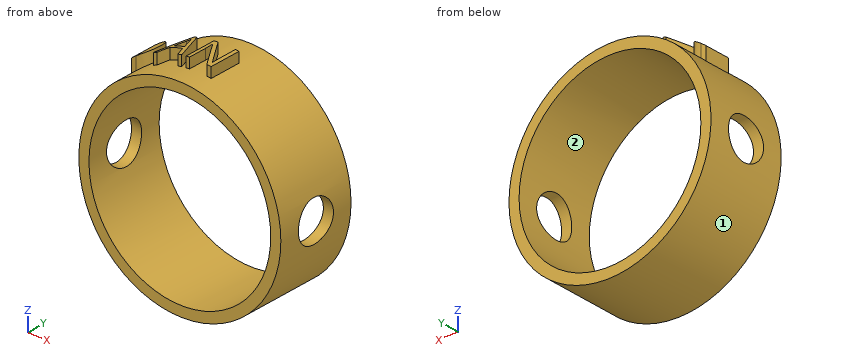
from build123d import *

# Parameters (mm, degrees)
F0_R     = 63.5
F0_R_2   = 57.15
F1_DEPTH = 50.8
F4_R     = 117.5833254056
F4_R_2   = 69.85
F5_DEPTH = 76.2
F7_R     = 12.7
F8_DEPTH = 76.2


with BuildPart() as f1:
    # F0 (on Front) → F1 (new body)
    with BuildSketch(Plane.XZ):
        Circle(F0_R)
        Circle(F0_R_2, mode=Mode.SUBTRACT)
    extrude(amount=F1_DEPTH)

    # F2 (on offset) → F3 (join, up to the next surface of F1)
    with BuildSketch(Plane.XY.offset(76.2)):
        with BuildLine():
            Line((5.7865704067, -37.8838032484), (8.454411462, -37.8838032484))
            Line((8.454411462, -37.8838032484), (8.454411462, -17.7693382623))
            Line((8.454411462, -17.7693382623), (6.2664296064, -17.7693382623))
            Line((6.2664296064, -17.7693382623), (6.2664296064, -29.3123733233))
            add(Edge.make_bspline(
                [(6.3368676541, -32.1959308995), (6.2400153385, -30.1796417852), (6.2664296064, -29.3123733233)],
                knots=[0, 0, 0, 1, 1, 1], degree=2))
            add(Edge.make_bspline(
                [(6.4601342375, -34.5820197642), (6.4337199696, -34.2122200139), (6.3368676541, -32.1959308995)],
                knots=[0, 0, 0, 1, 1, 1], degree=2))
            Line((6.4601342375, -34.5820197642), (6.350074788, -34.5820197642))
            Line((6.350074788, -34.5820197642), (-4.6162487577, -17.7693382623))
            Line((-4.6162487577, -17.7693382623), (-7.2576755451, -17.7693382623))
            Line((-7.2576755451, -17.7693382623), (-7.2576755451, -37.8838032484))
            Line((-7.2576755451, -37.8838032484), (-5.0961079574, -37.8838032484))
            Line((-5.0961079574, -37.8838032484), (-5.0961079574, -26.4508276369))
            add(Edge.make_bspline(
                [(-5.3162268563, -21.0050860769), (-5.0961079574, -23.9766912127), (-5.0961079574, -26.4508276369)],
                knots=[0, 0, 0, 1, 1, 1], degree=2))
            Line((-5.3162268563, -21.0050860769), (-5.2061674069, -21.0050860769))
            Line((-5.2061674069, -21.0050860769), (5.7865704067, -37.8838032484))
        make_face()
        Polygon((-14.9486298744, -31.4871480449), (-12.4436768043, -37.8838032484), (-10.0223689159, -37.8838032484), (-17.9334421442, -17.6856930807), (-19.9013051008, -17.6856930807), (-27.8519997309, -37.8838032484), (-25.4835203782, -37.8838032484), (-23.009383954, -31.4871480449), align=None)
        with BuildLine():
            Line((-18.0170873258, -23.1490441527), (-15.6750222409, -29.382811371))
            Line((-15.6750222409, -29.382811371), (-22.1817368939, -29.382811371))
            Line((-22.1817368939, -29.382811371), (-19.8176599192, -23.1490441527))
            add(Edge.make_bspline(
                [(-18.9503914573, -20.2478770645), (-19.2541555379, -21.5685904582), (-19.8176599192, -23.1490441527)],
                knots=[0, 0, 0, 1, 1, 1], degree=2))
            add(Edge.make_bspline(
                [(-18.0170873258, -23.1490441527), (-18.4705322576, -21.9648044763), (-18.9503914573, -20.2478770645)],
                knots=[0, 0, 0, 1, 1, 1], degree=2))
        make_face(mode=Mode.SUBTRACT)
        with BuildLine():
            add(Edge.make_bspline(
                [(-34.1540038078, -33.8050000509), (-32.0474659448, -31.7468883457), (-32.0474659448, -27.7187124949)],
                knots=[0, 0, 0, 1, 1, 1], degree=2))
            add(Edge.make_bspline(
                [(-32.0474659448, -27.7187124949), (-32.0474659448, -23.7829865817), (-34.0219324684, -21.7887093572)],
                knots=[0, 0, 0, 1, 1, 1], degree=2))
            add(Edge.make_bspline(
                [(-34.0219324684, -21.7887093572), (-35.996398992, -19.7944321327), (-39.8925035034, -19.7944321327)],
                knots=[0, 0, 0, 1, 1, 1], degree=2))
            Line((-39.8925035034, -19.7944321327), (-43.2911393032, -19.7944321327))
            Line((-43.2911393032, -19.7944321327), (-43.2911393032, -35.863111756))
            Line((-43.2911393032, -35.863111756), (-40.4428007508, -35.863111756))
            add(Edge.make_bspline(
                [(-40.4428007508, -35.863111756), (-36.2605416707, -35.863111756), (-34.1540038078, -33.8050000509)],
                knots=[0, 0, 0, 1, 1, 1], degree=2))
        make_face()
    extrude(until=Until.NEXT, dir=(0, 0, -1))

    # F4 (on Front) → F5 (cut, symmetric)
    with BuildSketch(Plane.XZ):
        with Locations((3.9105862379, 0.7332265377)):
            Circle(F4_R)
        Circle(F4_R_2, mode=Mode.SUBTRACT)
    extrude(amount=F5_DEPTH, both=True, mode=Mode.SUBTRACT)

    # F7 (on Right) → F8 (cut, symmetric)
    with BuildSketch(Plane.YZ):
        with Locations((-25.4, 0)):
            Circle(F7_R)
    extrude(amount=F8_DEPTH, both=True, mode=Mode.SUBTRACT)


solid = f1.part
For this review, take the finished solid that the model builds, in its own axes (mm). Face numbers are marked on the shaded views. Round coordinates to 2 decimals unless told otherwise and drop trailing zeros. Loops run counter-clockwise (first coordinate to the right, second up) from the corner with the lowest first, then second, coordinate; pieces in that order, holes last. Notation, with made-up numbers: (29.5, 37.25) - (63.5, 37.25) arc R22 cw to (63.5, 76.25) - close; hole circle Ø10 at (3.5, -33.5). An arc over 180 degrees is marked (long way). Put each result on its own line as item: value. Start each with the question number.
1. Consider section B-B on x = 0. State the section outline as (y, z) points, plus the area to 3 significant figures.
2. Consider section D-D on x = -53. State the section outline as (y, z) points (3 decimals), plus the area to 3 significant figures.
3. For probe 1 along Y at (x, z) = (59.5, 0); probe 2 along Z at (x, y) = (0, -11); probe 3 along X at (y, z) = (-13, 53) (3 decimals), list the stretches that pass through material, from the lowest coordinate up. Write a range as [from, to].
4. Insertion check: P1, Ø2, axis at x = 7.5, z = 65.5, coming from the -Y side; P2, Ø5, axis at y = -24, z = 66, coming from the -X side; P3, Ø4, axis at y = -8.5, z = -37, coming from the +X side; P4, Ø20.5, axis at y = -25.4, z = 0, coming from the +X side. Each pin has a flat end and moves straight along its axis. Give the tip position at first contact, or say it passes through.
5. Consider section A-A on z = 0. State the section outline as (x, y) points, plus the area to 3 significant figures.
6. Consider section C-C on y = -4. State the section outline as (x, z) points, plus the area to 3 significant figures.
7. Mouldability with a two-part tool opening along Z and no side actions: class the marked faces 1 and 2 as +Z half, -Z half, draft (parallel to the pull), parting line (faces both ways), or undercut.
Result sheet:
1. outline: (-50.8, -63.5) - (0, -63.5) - (0, -57.15) - (-50.8, -57.15) - close; (-50.8, 57.15) - (0, 57.15) - (0, 63.5) - (-24.85, 63.5) - (-24.85, 69.85) - (-29, 69.85) - (-29, 63.5) - (-50.8, 63.5) - close
1. area: 672 mm^2
2. outline: (-50.8, -34.975) - (0, -34.975) - (0, -21.38) - (-50.8, -21.38) - close; (-50.8, 21.38) - (0, 21.38) - (0, 34.975) - (-50.8, 34.975) - close
2. area: 1,380 mm^2
3. probe 1: [-50.8, -38.1], [-12.7, 0]
3. probe 2: [-63.5, -57.15], [57.15, 63.5]
3. probe 3: [-34.975, -21.38], [21.38, 34.975]
4. P1: y = -37.88
4. P2: x = -23.37
4. P3: x = 52.98
4. P4: through
5. outline: (-63.5, -50.8) - (-57.15, -50.8) - (-57.15, -38.1) - (-63.5, -38.1) - close; (-63.5, -12.7) - (-57.15, -12.7) - (-57.15, 0) - (-63.5, 0) - close; (57.15, -50.8) - (63.5, -50.8) - (63.5, -38.1) - (57.15, -38.1) - close; (57.15, -12.7) - (63.5, -12.7) - (63.5, 0) - (57.15, 0) - close
5. area: 323 mm^2
6. outline: circle Ø127 at (0, 0); hole circle Ø114.3 at (0, 0)
6. area: 2,410 mm^2
7. face 1: parting line
7. face 2: undercut
